from build123d import *

# Parameters (mm, degrees)
SKETCH1_W           = 320.802
SKETCH1_H           = 152.4
BOSS_EXTRUDE1_DEPTH = 0.79375
SKETCH2_W           = 13.0175
SKETCH2_H           = 12.7
SKETCH2_W_2         = 26.035
SKETCH2_W_3         = 2.9845
CUT_EXTRUDE1_DEPTH  = 1.79375
SKETCH3_R           = 2.413
CUT_EXTRUDE2_DEPTH  = 1.79375


with BuildPart() as part:
    # Sketch1 → Boss-Extrude1 (new body)
    with BuildSketch(Plane.XY):
        with Locations((160.401, 76.2)):
            Rectangle(SKETCH1_W, SKETCH1_H)
    extrude(amount=BOSS_EXTRUDE1_DEPTH)

    # Sketch2 → Cut-Extrude1 (cut, through all)
    with BuildSketch(Plane.XY.offset(0.79375)):
        with Locations((314.29325, 146.05)):
            Rectangle(SKETCH2_W, SKETCH2_H)
        with Locations((270.002, 146.05)):
            Rectangle(SKETCH2_W_2, SKETCH2_H)
        with Locations((219.202, 146.05)):
            Rectangle(SKETCH2_W_2, SKETCH2_H)
        with Locations((168.402, 146.05)):
            Rectangle(SKETCH2_W_2, SKETCH2_H)
        with Locations((117.602, 146.05)):
            Rectangle(SKETCH2_W_2, SKETCH2_H)
        with Locations((66.802, 146.05)):
            Rectangle(SKETCH2_W_2, SKETCH2_H)
        with Locations((16.002, 146.05)):
            Rectangle(SKETCH2_W_2, SKETCH2_H)
        with Locations((1.49225, 146.05)):
            Rectangle(SKETCH2_W_3, SKETCH2_H)
        with Locations((1.49225, 6.35)):
            Rectangle(SKETCH2_W_3, SKETCH2_H)
        with Locations((16.002, 6.35)):
            Rectangle(SKETCH2_W_2, SKETCH2_H)
        with Locations((66.802, 6.35)):
            Rectangle(SKETCH2_W_2, SKETCH2_H)
        with Locations((117.602, 6.35)):
            Rectangle(SKETCH2_W_2, SKETCH2_H)
        with Locations((168.402, 6.35)):
            Rectangle(SKETCH2_W_2, SKETCH2_H)
        with Locations((219.202, 6.35)):
            Rectangle(SKETCH2_W_2, SKETCH2_H)
        with Locations((270.002, 6.35)):
            Rectangle(SKETCH2_W_2, SKETCH2_H)
        with Locations((314.29325, 6.35)):
            Rectangle(SKETCH2_W, SKETCH2_H)
    extrude(amount=-CUT_EXTRUDE1_DEPTH, mode=Mode.SUBTRACT)

    # Sketch3 → Cut-Extrude2 (cut, through all)
    with BuildSketch(Plane.XY.offset(0.79375)):
        with Locations((41.402, 146.05)):
            Circle(SKETCH3_R)
        with Locations((92.202, 146.05)):
            Circle(SKETCH3_R)
        with Locations((143.002, 146.05)):
            Circle(SKETCH3_R)
        with Locations((193.802, 146.05)):
            Circle(SKETCH3_R)
        with Locations((244.602, 146.05)):
            Circle(SKETCH3_R)
        with Locations((295.402, 146.05)):
            Circle(SKETCH3_R)
        with Locations((92.202, 6.35)):
            Circle(SKETCH3_R)
        with Locations((143.002, 6.35)):
            Circle(SKETCH3_R)
        with Locations((193.802, 6.35)):
            Circle(SKETCH3_R)
        with Locations((244.602, 6.35)):
            Circle(SKETCH3_R)
        with Locations((295.402, 6.35)):
            Circle(SKETCH3_R)
        with Locations((41.402, 6.35)):
            Circle(SKETCH3_R)
    extrude(amount=-CUT_EXTRUDE2_DEPTH, mode=Mode.SUBTRACT)


solid = part.part
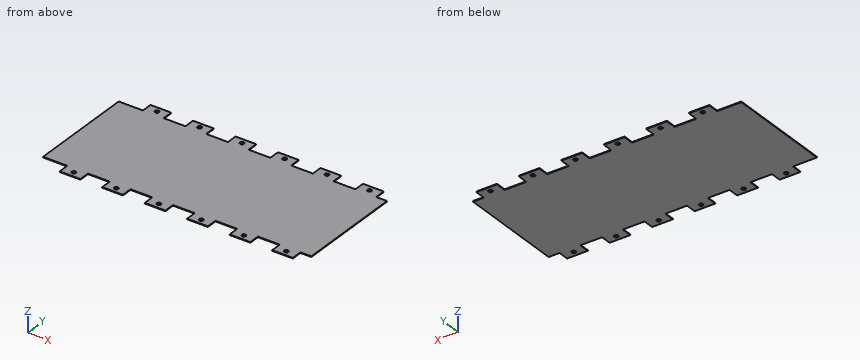
Geometry: final body of the model. Coordinates: model frame, mm. Round coordinates to 2 decimals unless told otherwise and drop trailing zeros. Loops run counter-clockwise (first coordinate to the right, second up) from the corner with the lowest first, then second, coordinate; pieces in that order, holes last. Notation, with made-up numbers: M -10.5,74.25 L 18.5,74.25 A12 ccw 18.5,89.25 Z; hole C -21,5 d5. An arc over 180 degrees is marked long. Put each result on its own line as item: value. Start each with the question number.
(1) Section query B-B (x = 227). Return loops of the section in (y, z).
(2) Material intervals for line 1 along X through (y, z) = (11.5, 0.35); line 2 along Y through (x, z) = (195, 0.05); line 3 along Y through (x, z) = (168, 0.1), sorted ascending. Write a range as [from, to].
(3) Section query A-A (z = 0.2). State how many separate pieces and enclosed holes the cut face has, then the cut area to 3 significant figures.
Findings below:
1. outline: M 12.7,0 L 139.7,0 L 139.7,0.79 L 12.7,0.79 Z
2. line 1: x = [29.02, 53.78], [79.82, 104.58], [130.62, 155.38], [181.42, 206.18], [232.22, 256.98], [283.02, 307.78]
2. line 2: y = [0, 4.26], [8.44, 143.96], [148.14, 152.4]
2. line 3: y = [12.7, 139.7]
3. separate pieces: 1
3. enclosed holes: 12
3. area: 44,300 mm2
